```python
from build123d import *

# Parameters (mm, degrees)
SKETCH1_R           = 57.75
SKETCH1_R_2         = 52.75
BOSS_EXTRUDE1_DEPTH = 750
FILLET1_R           = 2
FILLET2_R           = 2


with BuildPart() as part:
    # Sketch1 → Boss-Extrude1 (new body)
    with BuildSketch(Plane(origin=(0, 0, 0), x_dir=(0, 0, -1), z_dir=(1, 0, 0))):
        Circle(SKETCH1_R)
        Circle(SKETCH1_R_2, mode=Mode.SUBTRACT)
    extrude(amount=BOSS_EXTRUDE1_DEPTH)

    # Fillet1
    fillet1_edges = [part.edges().sort_by_distance(p)[0] for p in [
        (750, 0, 57.75),
        (750, 0, 52.75),
    ]]
    fillet(fillet1_edges, radius=FILLET1_R)

    # Fillet2
    fillet2_edges = [part.edges().sort_by_distance(p)[0] for p in [
        (0, 0, 57.75),
        (0, 0, 52.75),
    ]]
    fillet(fillet2_edges, radius=FILLET2_R)


solid = part.part
```
Geometry: final body of the model. Coordinates: model frame, mm. Round coordinates to 2 decimals unless told otherwise and drop trailing zeros. Loops run counter-clockwise (first coordinate to the right, second up) from the corner with the lowest first, then second, coordinate; pieces in that order, holes last. Notation, with made-up numbers: (82.25, 50) -> (141.25, 50) arc R15 ccw to (141.25, 63) -> close; hole circle Ø1 at (67, 59). An arc over 180 degrees is marked (long way). Use one line per item in the form item = value. Start each with the question number.
1) First-contact query: P1, Ø8, axis at x = 394, y = 31, coming from the -Z side; P2, Ø10, axis at x = 554, z = 10.5, coming from the +Y side; P3, Ø4, axis at x = 153.5, z = 13, coming from the +Y side. Flat tips, straight axial feed; report the tip coordinate or a pass-through.
2) Section C-C on x = 663. Output: boundary loops of the cut face in (y, z).
3) Line query: L1, parallel to Y at x = 547.5, z = 0; L2, parallel to Z at x = 570, y = -11; L3, parallel to Z at x = 346, y = -33. Output: solid intervals per line, ascending.
4) Section A-A on y = 0. Output: boundary loops of the cut face in (x, z), then the cut area to 3 significant figures.
5) Draft query along Y for faces 1 (the flat face through (0, -37, -41)), 2 (the cylindrical face through (369.78, 52.3, 6.87)), 3 (the cylindrical face through (369.78, -35.14, 45.83)). Return one class per face: released by +Y, released by -Y, zero draft, split by the parting line, or undercut.
Response:
q1.P1 = -51.05
q1.P2 = 57.49
q1.P3 = 56.69
q2.outline = circle Ø115.5 at (0, 0); hole circle Ø105.5 at (0, 0)
q3.L1 = -57.75 to -52.75, 52.75 to 57.75
q3.L2 = -56.69 to -51.59, 51.59 to 56.69
q3.L3 = -47.39 to -41.15, 41.15 to 47.39
q4.outline = (0, -55.75) arc R2 ccw to (2, -57.75) -> (748, -57.75) arc R2 ccw to (750, -55.75) -> (750, -54.75) arc R2 ccw to (748, -52.75) -> (2, -52.75) arc R2 ccw to (0, -54.75) -> close; (0, 54.75) arc R2 ccw to (2, 52.75) -> (748, 52.75) arc R2 ccw to (750, 54.75) -> (750, 55.75) arc R2 ccw to (748, 57.75) -> (2, 57.75) arc R2 ccw to (0, 55.75) -> close
q4.area = 7,490 mm^2
q5.face_1 = zero draft
q5.face_2 = undercut
q5.face_3 = split by the parting line
